from build123d import *

# Parameters (mm, degrees)
SKETCH2_R          = 25
SKETCH2_R_2        = 20
CUT_EXTRUDE5_DEPTH = 30
CUT_EXTRUDE6_DEPTH = 20


with BuildPart() as part:
    # Sketch3 → Revolve3 (revolve)
    with BuildSketch(Plane(origin=(0, 0, 0), x_dir=(0, 0, -1), z_dir=(1, 0, 0)), mode=Mode.PRIVATE) as revolve3_sk:
        Polygon((0, 0), (14.7, 0), (14.7, 4), (12.35, 15), (12.35, 20), (2.35, 20), (2.35, 15), (0, 4), align=None)
    revolve(revolve3_sk.sketch.rotate(Axis((0, 0, 0), (0, 0, -1)), 90), axis=Axis((0, 0, 0), (0, 0, -1)))

    # Sketch2 → Cut-Extrude5 (cut)
    with BuildSketch(Plane.XY):
        Circle(SKETCH2_R)
        Circle(SKETCH2_R_2, mode=Mode.SUBTRACT)
        with BuildLine():
            ThreePointArc((-12.513625189, -8.270984502), (-13.858192988, -5.740251485), (-14.696938457, -3))
            Line((-14.696938457, -3), (-19.773719933, -3))
            ThreePointArc((-19.773719933, -3), (-18.47759065, -7.653668647), (-16.103451798, -11.860811111))
            Line((-16.103451798, -11.860811111), (-12.513625189, -8.270984502))
        make_face()
        with BuildLine():
            ThreePointArc((-14.696938457, 3), (-13.858192988, 5.740251485), (-12.513625189, 8.270984502))
            Line((-12.513625189, 8.270984502), (-16.103451798, 11.860811111))
            ThreePointArc((-16.103451798, 11.860811111), (-18.47759065, 7.653668647), (-19.773719933, 3))
            Line((-19.773719933, 3), (-14.696938457, 3))
        make_face()
        with BuildLine():
            ThreePointArc((-8.270984502, 12.513625189), (-5.740251485, 13.858192988), (-3, 14.696938457))
            Line((-3, 14.696938457), (-3, 19.773719933))
            ThreePointArc((-3, 19.773719933), (-7.653668647, 18.47759065), (-11.860811111, 16.103451798))
            Line((-11.860811111, 16.103451798), (-8.270984502, 12.513625189))
        make_face()
        with BuildLine():
            Line((3, 19.773719933), (3, 14.696938457))
            ThreePointArc((3, 14.696938457), (5.740251485, 13.858192988), (8.270984502, 12.513625189))
            Line((8.270984502, 12.513625189), (11.860811111, 16.103451798))
            ThreePointArc((11.860811111, 16.103451798), (7.653668647, 18.47759065), (3, 19.773719933))
        make_face()
        with BuildLine():
            Line((16.103451798, 11.860811111), (12.513625189, 8.270984502))
            ThreePointArc((12.513625189, 8.270984502), (13.858192988, 5.740251485), (14.696938457, 3))
            Line((14.696938457, 3), (19.773719933, 3))
            ThreePointArc((19.773719933, 3), (18.47759065, 7.653668647), (16.103451798, 11.860811111))
        make_face()
        with BuildLine():
            ThreePointArc((16.103451798, -11.860811111), (18.47759065, -7.653668647), (19.773719933, -3))
            Line((19.773719933, -3), (14.696938457, -3))
            ThreePointArc((14.696938457, -3), (13.858192988, -5.740251485), (12.513625189, -8.270984502))
            Line((12.513625189, -8.270984502), (16.103451798, -11.860811111))
        make_face()
        with BuildLine():
            ThreePointArc((3, -19.773719933), (7.653668647, -18.47759065), (11.860811111, -16.103451798))
            Line((11.860811111, -16.103451798), (8.270984502, -12.513625189))
            ThreePointArc((8.270984502, -12.513625189), (5.740251485, -13.858192988), (3, -14.696938457))
            Line((3, -14.696938457), (3, -19.773719933))
        make_face()
        with BuildLine():
            ThreePointArc((-3, -14.696938457), (-5.740251485, -13.858192988), (-8.270984502, -12.513625189))
            Line((-8.270984502, -12.513625189), (-11.860811111, -16.103451798))
            ThreePointArc((-11.860811111, -16.103451798), (-7.653668647, -18.47759065), (-3, -19.773719933))
            Line((-3, -19.773719933), (-3, -14.696938457))
        make_face()
    extrude(amount=-CUT_EXTRUDE5_DEPTH, mode=Mode.SUBTRACT)

    # Sketch4 → Cut-Extrude6 (cut)
    with BuildSketch(Plane.XY):
        with BuildLine():
            Line((1.089724736, -2.25), (1.089724736, 2.25))
            ThreePointArc((1.089724736, 2.25), (-2.5, 0), (1.089724736, -2.25))
        make_face()
    extrude(amount=-CUT_EXTRUDE6_DEPTH, mode=Mode.SUBTRACT)


solid = part.part
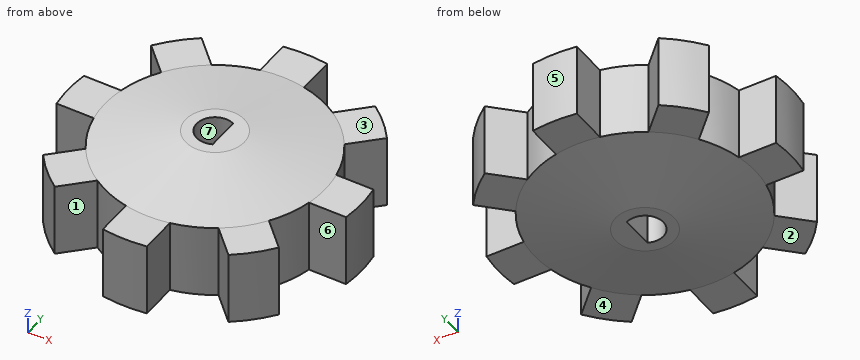
CAD build for the part. Positions are in the model's coordinates, mm. Face numbers are marked on the shaded views. A direction names the side the tool comes from. Give positions to 0.01 mm unless a question says otherwise; leave off trailing zeros. Loops run counter-clockwise (first coordinate to the right, second up) from the corner with the lowest first, then second, coordinate; pieces in that order, holes last. Notation, with made-up numbers: M 24,-26 L 74,-26 A24 cw 74,-8 Z; hole C 28,70.5 d1. An arc over 180 degrees is marked long. Write each question's results on one line, items separated by ' | '.
Q1. Band-saw the part on B-B on x = 0. Write the cut outline in (y, z), and give its area (3 significant figures).
Geometry check:
outline: M -20,-12.35 L -15,-12.35 L -4,-14.7 L -2.5,-14.7 L -2.5,0 L -4,0 L -15,-2.35 L -20,-2.35 Z; M 2.5,-14.7 L 4,-14.7 L 15,-12.35 L 20,-12.35 L 20,-2.35 L 15,-2.35 L 4,0 L 2.5,0 Z | area: 416 mm²
Q2. Band-saw the part on A-A on y = 0. Write the cut outline in (x, z), and give its area (3 significant figures).
Geometry check:
outline: M -20,-12.35 L -15,-12.35 L -4,-14.7 L -2.5,-14.7 L -2.5,0 L -4,0 L -15,-2.35 L -20,-2.35 Z; M 1.09,-14.7 L 4,-14.7 L 15,-12.35 L 20,-12.35 L 20,-2.35 L 15,-2.35 L 4,0 L 1.09,0 Z | area: 437 mm²
Q3. Mould opens along X. For the marked faces 5, 6 and 7 say: pulls with the +X half, pulls with the -X half, needs draft (parallel to the pull), parting line crosses it, or undercut.
Geometry check:
face 5: parting line crosses it | face 6: needs draft | face 7: undercut
Q4. Probe probe 1 along Y at (x, z) = (0, -11.5); probe 2 along X at (y, z) = (0, -5); probe 3 along X at (y, z) = (13.5, -7.5). List the from-to ranges inside material, lowest first.
Geometry check:
probe 1: y = -20 to -2.5, 2.5 to 20 | probe 2: x = -20 to -2.5, 1.09 to 20 | probe 3: x = -14.76 to -9.26, -6.54 to 6.54, 9.26 to 14.76
Q5. Which spindle directions (+Z, -Z, +X, -X, +Y, -Y) get a long thin tool onto all of the face, cutting with end or side? Do the marked faces 1, 2, 3 and 4. Say none if no direction does.
Geometry check:
face 1: +Z, -Z, -Y | face 2: -Z, -X, -Y | face 3: +Z, +X, +Y | face 4: -Z, +X, -Y
Q6. Band-saw the part on D-D on y = -14. Give the number of separate pieces and of enclosed holes in the cut face, and give its area (3 significant figures).
Geometry check:
separate pieces: 3 | enclosed holes: 0 | area: 201 mm²
Q7. Flat gauge pins, fed straight in: P1, Ø1.6, axis at x = -18.5, y = 0, coming from the -Z side; P2, Ø4, axis at y = -18, z = -8, coming from the +X side; P3, Ø3, axis at x = -1, z = -3, coming from the +Y side; P4, Ø6, axis at x = -1.5, y = -18.5, coming from the +Z side. Where does each tip first touch, or does it go through?
Geometry check:
P1: stops at z = -12.35 | P2: stops at x = 12 | P3: stops at y = 20 | P4: stops at z = -2.35
